from build123d import *

# Parameters (mm, degrees)
SKETCH005_W     = 34
SKETCH005_H     = 34
PAD005_DEPTH    = 3
SKETCH006_W     = 3
SKETCH006_H     = 34
PAD006_DEPTH    = 31
FILLET_R        = 3
FILLET001_R     = 5
SKETCH007_R     = 1.5
SKETCH007_R_2   = 3.6
POCKET_DEPTH    = 5
FILLET002_R     = 3
SKETCH008_R     = 1.5
SKETCH008_R_2   = 3.5
POCKET001_DEPTH = 5
FILLET003_R     = 3


with BuildPart() as part:
    # Sketch005 → Pad005 (new body)
    with BuildSketch(Plane.XY):
        with Locations((-37, 17)):
            Rectangle(SKETCH005_W, SKETCH005_H)
    extrude(amount=PAD005_DEPTH)

    # Sketch006 (on Face6 of Pad005) → Pad006 (join)
    with BuildSketch(Plane.XY.offset(3)):
        with Locations((-52.5, 17)):
            Rectangle(SKETCH006_W, SKETCH006_H)
    extrude(amount=PAD006_DEPTH)

    # Fillet
    fillet_edges = [part.edges().sort_by_distance(p)[0] for p in [
        (-51, 17, 3),
    ]]
    fillet(fillet_edges, radius=FILLET_R)

    # Fillet001
    fillet001_edges = [part.edges().sort_by_distance(p)[0] for p in [
        (-54, 17, 0),
    ]]
    fillet(fillet001_edges, radius=FILLET001_R)

    # Sketch007 (on Face6 of Fillet001) → Pocket (cut)
    with BuildSketch(Plane.XY.offset(3)):
        with Locations((-33, 8.5)):
            Circle(SKETCH007_R)
        with Locations((-33, 25.5)):
            Circle(SKETCH007_R)
        with Locations((-33, 17)):
            Circle(SKETCH007_R_2)
    extrude(amount=-POCKET_DEPTH, mode=Mode.SUBTRACT)

    # Fillet002
    fillet002_edges = [part.edges().sort_by_distance(p)[0] for p in [
        (-20, 34, 1.5),
        (-20, 0, 1.5),
    ]]
    fillet(fillet002_edges, radius=FILLET002_R)

    # Sketch008 (on Face9 of Fillet002) → Pocket001 (cut)
    with BuildSketch(Plane.YZ.offset(-51)):
        with Locations((8.5, 21)):
            Circle(SKETCH008_R)
        with Locations((25.5, 21)):
            Circle(SKETCH008_R)
        with Locations((17, 21)):
            Circle(SKETCH008_R_2)
    extrude(amount=-POCKET001_DEPTH, mode=Mode.SUBTRACT)

    # Fillet003
    fillet003_edges = [part.edges().sort_by_distance(p)[0] for p in [
        (-52.5, 34, 34),
        (-52.5, 0, 34),
    ]]
    fillet(fillet003_edges, radius=FILLET003_R)


solid = part.part
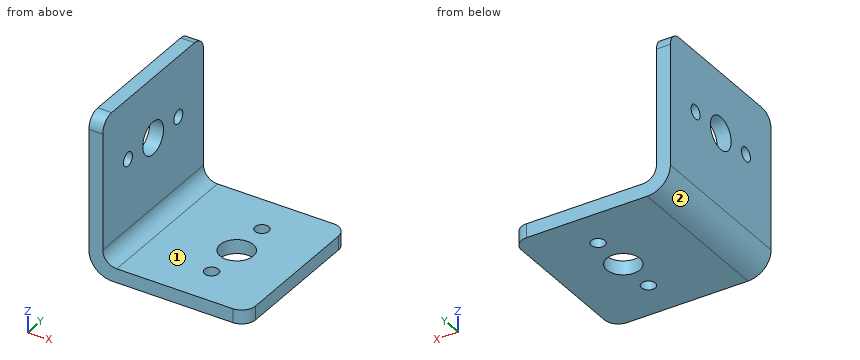
Here's how the part is built. I have some questions about the finished solid (model axes, mm). Face numbers are marked on the shaded views. A direction names the side the tool comes from. Coordinates: 2 decimals unless noted, no trailing zeros. Order: outer loops, then holes, each group sorted by start corner. A loop starts at its lowest first (then second) coordinate and runs counter-clockwise, first axis right, second up. Notation, with made-up numbers: (31, 66) -> (87, 66) arc R35 ccw to (87, 102) -> close; hole circle Ø5 at (-7, 9). An arc over 180 degrees is marked (long way). Answer in a Markdown table with one row per item.
(1) I want a section at D-D on y = 12.5. List the corners of the cut face in (x, z) for me, then the cut area to 3 significant figures.
Answer key:
| item | result |
|---|---|
| outline | (-54, 5) arc R5 ccw to (-49, 0) -> (-20, 0) -> (-20, 3) -> (-48, 3) arc R3 cw to (-51, 6) -> (-51, 34) -> (-54, 34) -> close |
| area | 192 mm^2 |
(2) On a 3-axis mill with a long thin cutter (end or side, diameter ignored), from which of +Z, -Z, +X, -X, +Y, -Y can I reach the whole of each face in a straight line? I mean the marked faces 1 and 2. Say none if no direction works.
Answer key:
| item | result |
|---|---|
| face 1 | +Z, +X, +Y, -Y |
| face 2 | -Z, -X, +Y, -Y |
(3) Please list where these lines run through material, in increasing order: probe 1 along Y at (x, z) = (-33, 1.45); probe 2 along X at (y, z) = (6, 32.5); probe 3 along Z at (x, y) = (-42, 2).
Answer key:
| item | result |
|---|---|
| probe 1 | 0 to 7, 10 to 13.4, 20.6 to 24, 27 to 34 |
| probe 2 | -54 to -51 |
| probe 3 | 0 to 3 |
(4) Will these pins go through, and if not, where does the flat tip stop? pin 1 Ø8.5 at (x, y) = (-33, 17) entering from +Z; pin 2 Ø12 at (y, z) = (23.5, 14.5) entering from +X.
Answer key:
| item | result |
|---|---|
| pin 1 | z = 3 |
| pin 2 | x = -51 |
(5) I want a section at A-A on z = 21. List the corners of the cut face in (x, y) for me.
Answer key:
| item | result |
|---|---|
| outline | (-54, 0) -> (-51, 0) -> (-51, 7) -> (-54, 7) -> close; (-54, 10) -> (-51, 10) -> (-51, 13.5) -> (-54, 13.5) -> close; (-54, 20.5) -> (-51, 20.5) -> (-51, 24) -> (-54, 24) -> close; (-54, 27) -> (-51, 27) -> (-51, 34) -> (-54, 34) -> close |
(6) I want a section at B-B on x = -33. List the corners of the cut face in (y, z) for me, then the cut area to 3 significant figures.
Answer key:
| item | result |
|---|---|
| outline | (0, 0) -> (7, 0) -> (7, 3) -> (0, 3) -> close; (10, 0) -> (13.4, 0) -> (13.4, 3) -> (10, 3) -> close; (20.6, 0) -> (24, 0) -> (24, 3) -> (20.6, 3) -> close; (27, 0) -> (34, 0) -> (34, 3) -> (27, 3) -> close |
| area | 62.4 mm^2 |
(7) I want a section at C-C on y = 25.5. List the corners of the cut face in (x, z) for me.
Answer key:
| item | result |
|---|---|
| outline | (-54, 5) arc R5 ccw to (-49, 0) -> (-34.5, 0) -> (-34.5, 3) -> (-48, 3) arc R3 cw to (-51, 6) -> (-51, 19.5) -> (-54, 19.5) -> close; (-54, 22.5) -> (-51, 22.5) -> (-51, 34) -> (-54, 34) -> close; (-31.5, 0) -> (-20, 0) -> (-20, 3) -> (-31.5, 3) -> close |
